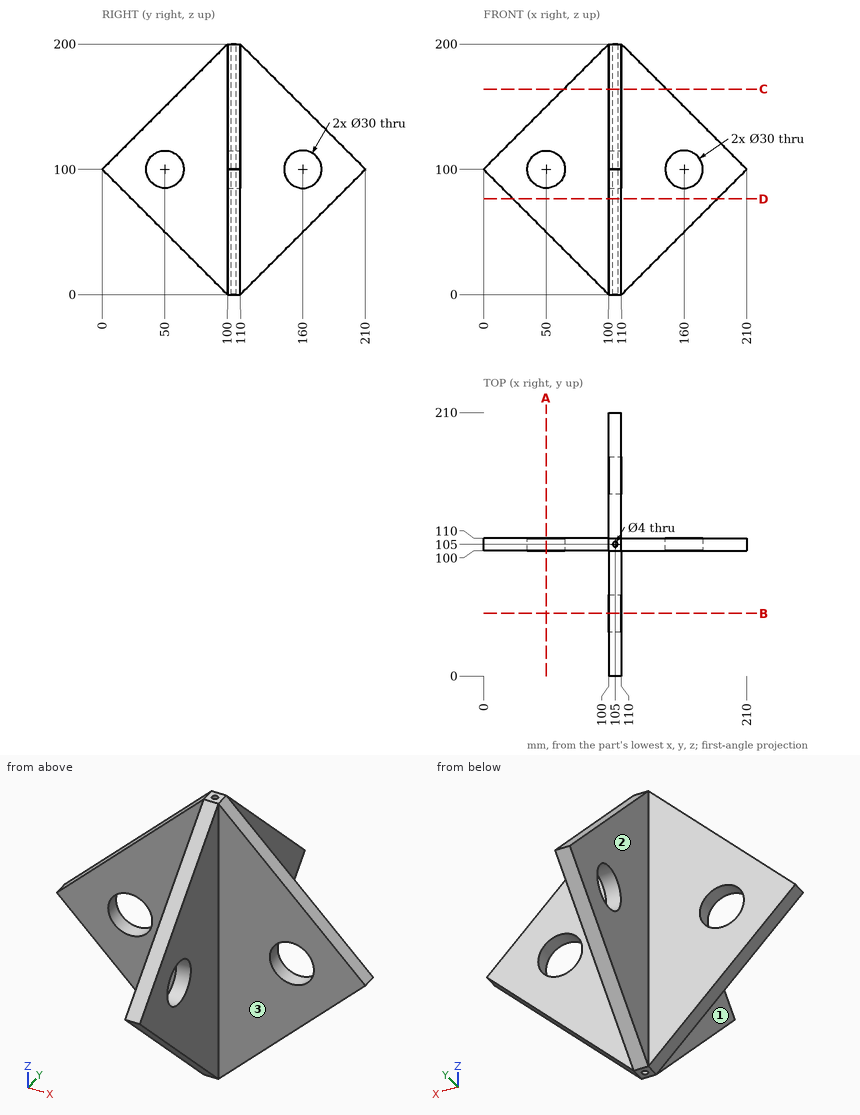
Answer from the drawing. Dimensions are ordinates in mm from the lowest x, y and z of the part. A direction names the side the tool comes from. Coordinates: 2 decimals unless noted, no trailing zeros. Order: outer loops, then holes, each group sorted by start corner. A loop starts at its lowest first (then second) coordinate and runs counter-clockwise, first axis right, second up. Notation, with made-up numbers: (76, -7.5) - (99, -7.5) arc R31 ccw to (99, 29.5) - close; hole circle Ø9 at (66.5, -38). An arc over 180 degrees is marked (long way). Put each result on its own line as item: value. Start each with the question number.
1) Find section D-D (z = 76.5). Give the vertices of the cut face in (x, y), plus the area to 3 significant figures.
2) Find the intervals of material crossed by line 1 (Y direction, x = 105, z = 93); line 2 (Y direction, x = 71, z = 95.5), in increasing order. Write a range as from..to.
3) Find section C-C (z = 164). Give the vertices of the cut face in (x, y).
4) Find section A-A (x = 50). Give the vertices of the cut face in (y, z), plus the area to 3 significant figures.
5) For the marked faces 1, 2 and 3, determine the directions among +Z, -Z, +X, -X, +Y, -Y from which every point of the face is accessible in a straight line to the end or side of a thin tool.
6) Flat-ended cylindrical pins translate along their axes: pin 1 (5 mm diameter, centred on y = 109.5, z = 62.5, fed in from +X); pin 2 (1 mm diameter, centred on y = 124, z = 146.5, fed in from +X); pin 3 (3.5 mm diameter, centred on x = 105, y = 105, fed in from +Z); pin 4 (5 mm diameter, centred on x = 23, z = 75.5, fed in from +Y). Find the tip coordinate at first contact, or state that the pin passes through.
Results list:
1. outline: (23.5, 100) - (100, 100) - (100, 23.5) - (110, 23.5) - (110, 100) - (186.5, 100) - (186.5, 110) - (110, 110) - (110, 186.5) - (100, 186.5) - (100, 110) - (23.5, 110) - close; hole circle Ø4 at (105, 105)
1. area: 3,150 mm^2
2. line 1: y = 7..36.73, 63.27..103, 107..146.73, 173.27..203
2. line 2: y = 100..110
3. outline: (64, 100) - (100, 100) - (100, 64) - (110, 64) - (110, 100) - (146, 100) - (146, 110) - (110, 110) - (110, 146) - (100, 146) - (100, 110) - (64, 110) - close; hole circle Ø4 at (105, 105)
4. outline: (100, 50) - (110, 50) - (110, 85) - (100, 85) - close; (100, 115) - (110, 115) - (110, 150) - (100, 150) - close
4. area: 700 mm^2
5. face 1: +Z, -Z, -X, -Y
5. face 2: +Z, -Z, -X, +Y
5. face 3: +Z, -Z, +X, -Y
6. pin 1: stops at x = 175
6. pin 2: stops at x = 110
6. pin 3: passes through
6. pin 4: stops at y = 110
